For this review, take the finished solid that the model builds, in its own axes (mm). A direction names the side the tool comes from. Give positions to 0.01 mm unless a question says otherwise; leave off trailing zeros. Write each loop counter-clockwise with the first axis right and the second up, starting at its lowest first coordinate (ties: lowest second). Pieces come first, ordered by that corner, then holes. Notation, with made-up numbers: (-16, -16) -> (17, -16) arc R23 cw to (17, -5) -> close; hole circle Ø2 at (63, 64.5). An arc over 180 degrees is marked (long way). Return JSON: item names as keys, results as strings.
from build123d import *

# Parameters (mm, degrees)
F0_W     = 3.1242
F0_H     = 3.175
F2_DEPTH = 3.175
F0_W_2   = 0.254
F0_W_3   = 6.35
F0_H_2   = 3.81
F4_W     = 3.175
F4_H     = 3.175
F5_DEPTH = 6.35
F6_W     = 6.35
F6_H     = 3.175
F7_DEPTH = 12.954
F9_DEPTH = 6.35


with BuildPart() as f1:
    # F0 (on Front) → F1 (revolve)
    with BuildSketch(Plane.XZ):
        Polygon((3.2258, 3.175), (0, 3.175), (0, 1.5875), (6.35, 0), (19.05, 0), (6.35, 3.175), (6.35, 6.35), (3.2258, 6.35), align=None)
        Polygon((3.2258, 9.525), (3.2258, 6.35), (6.35, 6.35), (6.35, 7.9375), (6.35, 9.525), align=None)
        Polygon((3.2258, 12.7), (3.2258, 9.525), (6.35, 9.525), (6.35, 11.1125), (6.35, 12.7), align=None)
        with Locations((4.7879, 14.2875)):
            Rectangle(F0_W, F0_H)
    revolve(axis=Axis((0, 0, 9.525), (0, 0, 1)))

    # F0 (on Front) → F2 (join, symmetric)
    with BuildSketch(Plane.XZ):
        Polygon((6.35, 7.9375), (6.35, 6.35), (42.1522888519, 19.3809674607), (42.1522888519, 20.9684674607), (39.5324932131, 20.0149398283), (10.0352127619, 9.2788077523), align=None)
        with BuildLine():
            Line((8.1232022233, 10.1703928286), (6.35, 9.525))
            Line((6.35, 9.525), (6.35, 7.9375))
            Line((6.35, 7.9375), (10.0352127619, 9.2788077523))
            ThreePointArc((10.0352127619, 9.2788077523), (8.8945541682, 9.3286099229), (8.1232022233, 10.1703928286))
        make_face()
        with BuildLine():
            Line((6.35, 11.1125), (6.35, 9.525))
            Line((6.35, 9.525), (8.1232022233, 10.1703928286))
            ThreePointArc((8.1232022233, 10.1703928286), (8.173004472, 11.3110514176), (9.014787429, 12.0824033048))
            Line((9.014787429, 12.0824033048), (6.35, 11.1125))
        make_face()
        Polygon((42.1522888519, 25.7309674607), (6.35, 12.7), (6.35, 11.1125), (9.014787429, 12.0824033048), (38.5120679189, 22.8185353949), (42.1522888519, 24.1434674607), align=None)
        Polygon((3.2258, 12.7), (3.2258, 9.525), (6.35, 9.525), (6.35, 11.1125), (6.35, 12.7), align=None)
        Polygon((3.2258, 9.525), (3.2258, 6.35), (6.35, 6.35), (6.35, 7.9375), (6.35, 9.525), align=None)
        with BuildLine():
            Line((42.1015425762, 22.5374973268), (42.1522888519, 22.5377925414))
            Line((42.1522888519, 22.5377925414), (42.1522888519, 24.1434674607))
            Line((42.1522888519, 24.1434674607), (38.5120679189, 22.8185353949))
            ThreePointArc((38.5120679189, 22.8185353949), (39.65272644, 22.7687331418), (40.4240783174, 21.9269502676))
            Line((40.4240783174, 21.9269502676), (40.5140425762, 21.9596945799))
            Line((40.5140425762, 21.9596945799), (42.1015425762, 22.5374973268))
        make_face()
        with BuildLine():
            Line((39.5324932131, 20.0149398283), (42.1522888519, 20.9684674607))
            Line((42.1522888519, 20.9684674607), (42.1522888519, 22.5377925414))
            Line((42.1522888519, 22.5377925414), (42.1015425762, 22.5374973268))
            Line((42.1015425762, 22.5374973268), (40.5140425762, 21.9596945799))
            Line((40.5140425762, 21.9596945799), (40.4240783174, 21.9269502676))
            ThreePointArc((40.4240783174, 21.9269502676), (40.4913793589, 21.6757793614), (40.5140425762, 21.4167376024))
            ThreePointArc((40.5140425762, 21.4167376024), (40.2442604638, 20.5610980533), (39.5324932131, 20.0149398283))
        make_face()
        Polygon((45.2764888519, 25.7309674607), (42.1522888519, 25.7309674607), (42.1522888519, 24.1434674607), (42.1522888519, 22.5377925414), (45.2764888519, 22.5559674607), align=None)
        Polygon((42.1522888519, 20.9684674607), (42.1522888519, 19.3809674607), (45.2764888519, 19.3809674607), (45.2764888519, 22.5559674607), (42.1522888519, 22.5377925414), align=None)
    extrude(amount=F2_DEPTH, both=True)



with BuildPart() as f2:
    # F0 (on Front) → F2, piece 2 (new body, symmetric)
    with BuildSketch(Plane.XZ):
        with Locations((54.9792888519, 17.7934674607)):
            Rectangle(F0_W_2, F0_H)
    extrude(amount=F2_DEPTH, both=True)

    # F0 (on Front) → F2, piece 3 (join, symmetric)
    with BuildSketch(Plane.XZ):
        Polygon((51.7280888519, 22.5559674607), (51.7280888519, 19.3809674607), (54.8522888519, 19.3809674607), (54.8522888519, 20.9684674607), (54.8522888519, 22.5559674607), align=None)
        Polygon((51.7280888519, 25.7309674607), (51.7280888519, 22.5559674607), (54.8522888519, 22.5559674607), (54.8522888519, 24.1434674607), (54.8522888519, 25.7309674607), align=None)
        Polygon((90.6545777039, 38.7619349214), (54.8522888519, 25.7309674607), (54.8522888519, 24.1434674607), (57.5170761795, 25.1133707286), (86.9693651328, 35.8331272386), (90.6545777039, 37.1744349214), align=None)
        with BuildLine():
            Line((54.8522888519, 24.1434674607), (54.8522888519, 22.5559674607))
            Line((54.8522888519, 22.5559674607), (56.6254910752, 23.2013602893))
            ThreePointArc((56.6254910752, 23.2013602893), (56.6752933011, 24.3420188294), (57.5170761795, 25.1133707286))
            Line((57.5170761795, 25.1133707286), (54.8522888519, 24.1434674607))
        make_face()
        with BuildLine():
            Line((54.8522888519, 22.5559674607), (54.8522888519, 20.9684674607))
            Line((54.8522888519, 20.9684674607), (58.5375015244, 22.3097751804))
            ThreePointArc((58.5375015244, 22.3097751804), (57.3968429771, 22.3595774037), (56.6254910752, 23.2013602893))
            Line((56.6254910752, 23.2013602893), (54.8522888519, 22.5559674607))
        make_face()
        Polygon((54.8522888519, 20.9684674607), (54.8522888519, 19.3809674607), (90.6545777039, 32.4119349214), (90.6545777039, 33.9994349214), (87.9897903763, 33.0295316535), (58.5375015244, 22.3097751804), align=None)
        with BuildLine():
            Line((87.9897903763, 33.0295316535), (90.6545777039, 33.9994349214))
            Line((90.6545777039, 33.9994349214), (90.6545777039, 35.5869349214))
            Line((90.6545777039, 35.5869349214), (88.8813754806, 34.9415420928))
            ThreePointArc((88.8813754806, 34.9415420928), (88.9486765221, 34.6903711866), (88.9713397394, 34.4313294276))
            ThreePointArc((88.9713397394, 34.4313294276), (88.7015576271, 33.5756898786), (87.9897903763, 33.0295316535))
        make_face()
        with BuildLine():
            Line((88.8813754806, 34.9415420928), (90.6545777039, 35.5869349214))
            Line((90.6545777039, 35.5869349214), (90.6545777039, 37.1744349214))
            Line((90.6545777039, 37.1744349214), (86.9693651328, 35.8331272386))
            ThreePointArc((86.9693651328, 35.8331272386), (88.1100236277, 35.7833249556), (88.8813754806, 34.9415420928))
        make_face()
        Polygon((90.6545777039, 33.9994349214), (90.6545777039, 32.4119349214), (97.0045777039, 32.4119349214), (97.0045777039, 38.7619349214), (90.6545777039, 38.7619349214), (90.6545777039, 37.1744349214), (90.6545777039, 35.5869349214), align=None)
        with Locations((93.8295777039, 40.6669349214)):
            Rectangle(F0_W_3, F0_H_2)
    extrude(amount=F2_DEPTH, both=True)


with BuildPart() as f1_1:
    add(f1.part)

    add(f2.part)  # F3 merges F2
    # F0 (on Front) → F3 (revolve)
    with BuildSketch(Plane.XZ):
        Polygon((45.2764888519, 16.2059674607), (42.1522888519, 16.2059674607), (42.1522888519, 14.6184674607), (48.5022888519, 14.6184674607), (48.5022888519, 16.2059674607), align=None)
        with Locations((43.7143888519, 17.7934674607)):
            Rectangle(F0_W, F0_H)
        Polygon((42.1522888519, 20.9684674607), (42.1522888519, 19.3809674607), (45.2764888519, 19.3809674607), (45.2764888519, 22.5559674607), (42.1522888519, 22.5377925414), align=None)
        Polygon((45.2764888519, 25.7309674607), (42.1522888519, 25.7309674607), (42.1522888519, 24.1434674607), (42.1522888519, 22.5377925414), (45.2764888519, 22.5559674607), align=None)
        with Locations((43.7143888519, 27.3184674607)):
            Rectangle(F0_W, F0_H)
    revolve(axis=Axis((48.5022888519, 0, 22.5559674607), (0, 0, 1)))

    # F4 (on Right) → F5 (cut)
    with BuildSketch(Plane.YZ):
        with Locations((-1.5875, 4.7625)):
            Rectangle(F4_W, F4_H)
        with Locations((1.5875, 4.7625)):
            Rectangle(F4_W, F4_H)
    extrude(amount=F5_DEPTH, mode=Mode.SUBTRACT)

    # F6 (on face) → F7 (cut)
    with BuildSketch(Plane.YZ.offset(55.1062888519)):
        with Locations((0, 17.7934674607)):
            Rectangle(F6_W, F6_H)
    extrude(amount=-F7_DEPTH, mode=Mode.SUBTRACT)

    # F8 (on face) → F9 (join)
    with BuildSketch(Plane.YZ.offset(97.0045777039)):
        Polygon((0, 41.9369349214), (-2.4077083333, 41.9369349214), (0, 40.6669349214), align=None)
        Polygon((2.4077083333, 41.9369349214), (0, 41.9369349214), (0, 40.6669349214), align=None)
        Polygon((0, 33.0469349214), (0, 34.3169349214), (-2.4077083333, 33.0469349214), align=None)
        Polygon((2.4077083333, 33.0469349214), (0, 34.3169349214), (0, 33.0469349214), align=None)
        Polygon((2.4077083333, 33.0469349214), (2.4077083333, 35.5869349214), (0, 34.3169349214), align=None)
        Polygon((2.4077083333, 35.5869349214), (0, 35.5869349214), (0, 34.3169349214), align=None)
        Polygon((0, 34.3169349214), (0, 35.5869349214), (-2.4077083333, 35.5869349214), align=None)
        Polygon((0, 34.3169349214), (-2.4077083333, 35.5869349214), (-2.4077083333, 33.0469349214), align=None)
        Polygon((0, 40.6669349214), (-2.4077083333, 39.3969349214), (0, 39.3969349214), align=None)
        Polygon((0, 40.6669349214), (-2.4077083333, 41.9369349214), (-2.4077083333, 39.3969349214), align=None)
        Polygon((2.4077083333, 39.3969349214), (0, 40.6669349214), (0, 39.3969349214), align=None)
        Polygon((2.4077083333, 41.9369349214), (0, 40.6669349214), (2.4077083333, 39.3969349214), align=None)
    extrude(amount=F9_DEPTH)


solid = f1_1.part
1. Add section C-C, the plane x = 94. State the section outline as (y, z) points (3 decimals), plus the area to 3 significant figures.
Results found:
{"outline": "(-3.175, 32.412) -> (3.175, 32.412) -> (3.175, 42.572) -> (-3.175, 42.572) -> close", "area": "64.5 mm²"}
2. Add section A-A, the plane z = 27. State the section outline as (x, y) points (3 decimals).
Results found:
{"outline": "circle Ø12.7 at (48.502, 0); (58.339, -3.175) -> (62.701, -3.175) -> (62.701, 3.175) -> (58.339, 3.175) -> close; (71.424, -3.175) -> (75.785, -3.175) -> (75.785, 3.175) -> (71.424, 3.175) -> close; hole circle Ø6.452 at (48.502, 0)"}
3. Add section B-B, the plane x = 80.5. State the section outline as (y, z) points (3 decimals), plus the area to 3 significant figures.
Results found:
{"outline": "(-3.175, 28.716) -> (3.175, 28.716) -> (3.175, 30.303) -> (-3.175, 30.303) -> close; (-3.175, 33.478) -> (3.175, 33.478) -> (3.175, 35.066) -> (-3.175, 35.066) -> close", "area": "20.2 mm²"}
4. To check wall thickness, follow probe 1 along Y at (x, z) = (0, 8); probe 2 along X at (y, z) = (0, 6); probe 3 along Z at (x, y) = (-4, -8). State the ranges of each line that lie inside material, in increasing order.
Results found:
{"probe 1": "y = -6.35 to -3.23, 3.23 to 6.35", "probe 2": "x = -6.35 to -3.23", "probe 3": "z = 0 to 2.53"}
5. For faces 4 (the flat face through (100, 0, 33.047)), 5 (the cylindrical face through (48.9, -3.2, 24.1)), 6 (the flat face through (100, 0, 39.397)), 7 (the flat face through (46, 3.175, 18)), 8 (the flat face through (24.502, -0.044, 19.307)), list the 3-axis set-ups (+Z, -Z, +X, -X, +Y, -Y) from which the entire face can be reached by the end or side of a thin tool; tool diameter is ignored.
Results found:
{"face 4": "-Z, +X, +Y, -Y", "face 5": "+Z", "face 6": "+X, +Y, -Y", "face 7": "+X", "face 8": "+Z, +Y, -Y"}
6. For pin 1 (18.5 mm diameter, centred on x = 71.5, z = 30.5, fed in from +Y) (3 decimals); pin 2 (1 mm diameter, centred on x = 46.5, z = 18.5, fed in from +Y); pin 3 (3 mm diameter, centred on x = -6.5, y = 1, fed in from +Z) (3 decimals), all flat-tipped, find the tip position at first contact; note any pin that passes through.
Results found:
{"pin 1": "stops at y = 3.175", "pin 2": "stops at y = 6.17", "pin 3": "stops at z = 15.875"}
7. The part is to be moulded in two halves that separate along Z. For faces 1 (the flat face through (94, 0, 42.572)), 2 (the flat face through (24.99, -0.04, 14.72)), 3 (the conical face through (-0.086, -0.388, 1.488)), say which applies: +Z half, -Z half, draft (parallel to the pull), parting line (faces both ways), or undercut.
Results found:
{"face 1": "+Z half", "face 2": "undercut", "face 3": "-Z half"}
